Drawing for the job (mm, zero at the part's lowest x, y, z). A direction names the side the tool comes from. Give positions to 0.01 mm unless a question says otherwise; leave off trailing zeros. Write each loop counter-clockwise with the first axis right and the second up, starting at its lowest first coordinate (ties: lowest second). Pieces come first, ordered by that corner, then holes. Notation, with made-up numbers: M 18,21.5 L 29,21.5 A13 ccw 29,30.5 Z; hole C 32,26.5 d8. An arc over 180 degrees is marked long. Use CSV: the item, a comma, the result in double quotes. Start each with the question number.
1. Band-saw the part on B-B, the plane x = 14. List the corners of the cut face in (y, z), then the cut area to 3 significant figures.
2. Mould opens along X. For the marked faces 4, 5, 6 and 7 say: pulls with the +X half, pulls with the -X half, needs draft (parallel to the pull), parting line crosses it, or undercut.
3. Band-saw the part on C-C, the plane y = 5.75. List the corners of the cut face in (x, z).
4. Drop flat-ended pins along their axis: pin 1 Ø15 at (x, z) = (28, 19) entering from -Y; pin 2 Ø3 at (y, z) = (2.5, 24.5) entering from -X; pin 3 Ø4 at (x, y) = (18, 3.5) entering from -Z; pin 4 Ø2 at (x, z) = (35, 4) entering from -Y. Give the stop position or say it passes through.
5. 3-axis set-ups, long thin cutter, end or side, ignore diameter. For the marked faces 1, 2 and 3: which of +Z, -Z, +X, -X, +Y, -Y reach the whole face in a straight line?
6. Band-saw the part on D-D, the plane x = 21.5. List the corners of the cut face in (y, z).
7. Band-saw the part on A-A, the plane z = 25.75. List the corners of the cut face in (x, y) (3 decimals), then the cut area to 3 significant figures.
8. Drill centre lines: line 1 along Y through (x, z) = (34.5, 4.25); line 2 along X through (y, z) = (5.25, 15.5); line 3 along Z through (x, y) = (14.5, 4.25). Where is each one in solid material? Low to high. Write a range as from..to.
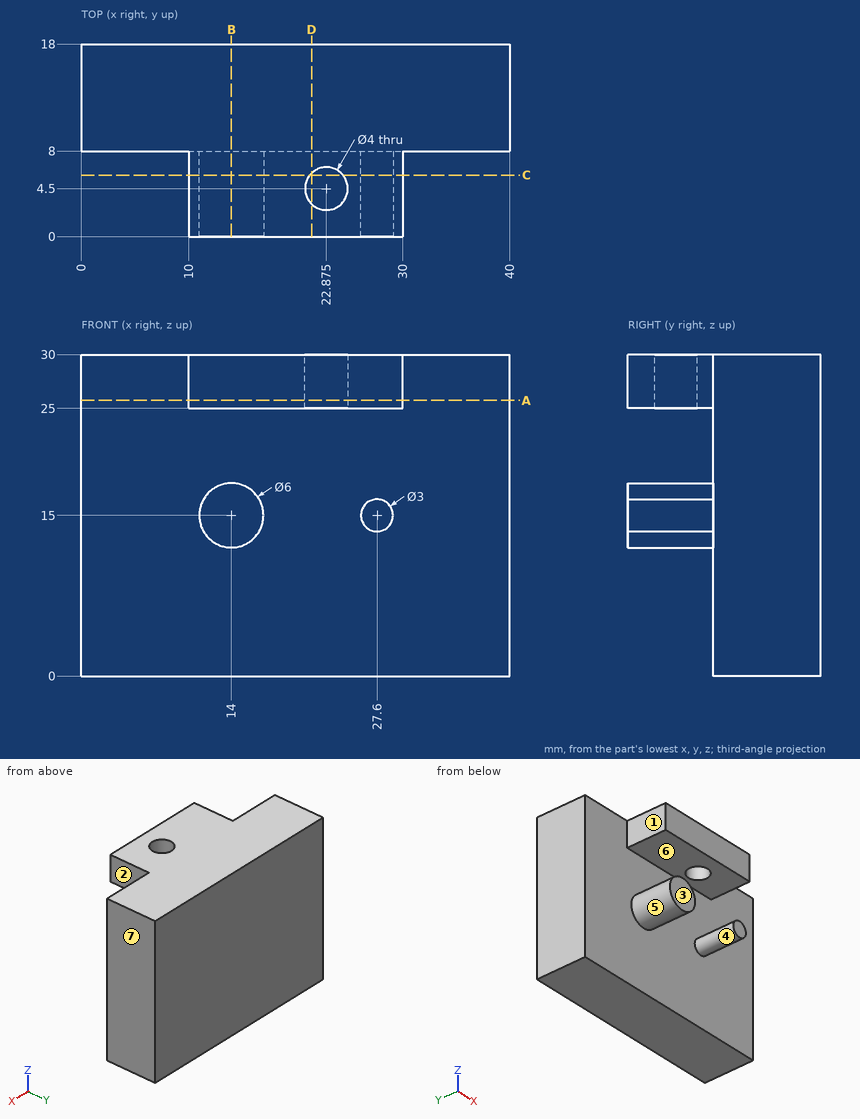
Output:
1,outline,"M 0,12 L 8,12 L 8,0 L 18,0 L 18,30 L 0,30 L 0,25 L 8,25 L 8,18 L 0,18 Z"
1,area,"388 mm²"
2,face 4,"undercut"
2,face 5,"undercut"
2,face 6,"needs draft"
2,face 7,"pulls with the +X half"
3,outline,"M 10,25 L 21.31,25 L 21.31,30 L 10,30 Z; C 14,15 d6; M 24.44,25 L 30,25 L 30,30 L 24.44,30 Z; C 27.6,15 d3"
4,pin 1,"stops at y = 0"
4,pin 2,"stops at x = 10"
4,pin 3,"stops at z = 12.76"
4,pin 4,"stops at y = 8"
5,face 1,"+Z, -Z, -X, -Y"
5,face 2,"+Z, -Z, +X, -Y"
5,face 3,"+Z, -Z, +X, -X, -Y"
6,outline,"M 0,25 L 3.05,25 L 3.05,30 L 0,30 Z; M 5.95,25 L 8,25 L 8,0 L 18,0 L 18,30 L 5.95,30 Z"
7,outline,"M 0,8 L 10,8 L 10,0 L 30,0 L 30,8 L 40,8 L 40,18 L 0,18 Z; hole C 22.875,4.5 d4"
7,area,"547 mm²"
8,line 1,"y = 8..18"
8,line 2,"x = 11.04..16.96, 26.19..29.01"
8,line 3,"z = 12.04..17.96, 25..30"
